```python
from build123d import *

# Parameters (mm, degrees)
ESQUISSE1_W                  = 90
ESQUISSE1_H                  = 25
BOSS_EXTRU_1_DEPTH           = 6
ESQUISSE2_W                  = 90
ESQUISSE2_H                  = 6
BOSS_EXTRU_2_DEPTH           = 40
ESQUISSE3_W                  = 40
ESQUISSE3_H                  = 6
BOSS_EXTRU_3_DEPTH           = 19
BOSS_EXTRU_4_DEPTH           = 6
ESQUISSE5_R                  = 2
ENL_V_MAT_EXTRU_1_DEPTH      = 157.783289926
ENL_V_MAT_EXTRU_2_DEPTH      = 160.25137362
ENL_V_MAT_EXTRU_2_DEPTH_BACK = 160.25137362
ESQUISSE6_R                  = 2
CHANFREIN1_SIZE              = 10
ESQUISSE7_R                  = 5
ENL_V_MAT_EXTRU_3_DEPTH      = 157.783289926
ESQUISSE8_R                  = 5
ENL_V_MAT_EXTRU_4_DEPTH      = 160.25137362
CHANFREIN3_SIZE              = 2.5
CONG_1_R                     = 10
CONG_2_R                     = 5


with BuildPart() as part:
    # Esquisse1 → Boss.-Extru.1 (new body)
    with BuildSketch(Plane.XY):
        with Locations((45, 12.5)):
            Rectangle(ESQUISSE1_W, ESQUISSE1_H)
    extrude(amount=BOSS_EXTRU_1_DEPTH)

    # Esquisse2 → Boss.-Extru.2 (add)
    with BuildSketch(Plane(origin=(90, 0, 0), x_dir=(0, 0, -1), z_dir=(1, 0, 0))):
        with Locations((-45, 3)):
            Rectangle(ESQUISSE2_W, ESQUISSE2_H)
    extrude(amount=BOSS_EXTRU_2_DEPTH)

    # Esquisse3 → Boss.-Extru.3 (add)
    with BuildSketch(Plane(origin=(0, 6, 0), x_dir=(1, 0, 0), z_dir=(0, 1, 0))):
        with Locations((110, -3)):
            Rectangle(ESQUISSE3_W, ESQUISSE3_H)
    extrude(amount=BOSS_EXTRU_3_DEPTH)

    # Esquisse4 → Boss.-Extru.4 (add)
    with BuildSketch(Plane.XZ):
        Polygon((0, 6), (90, 90), (90, 6), align=None)
    extrude(amount=-BOSS_EXTRU_4_DEPTH)

    # Esquisse5 → Enlèv. mat.-Extru.1 (cut, through all)
    with BuildSketch(Plane.XY.offset(6)):
        with Locations((45, 15.5)):
            Circle(ESQUISSE5_R)
        with Locations((15, 15.5)):
            Circle(ESQUISSE5_R)
        with Locations(Location((75, 15.5, 0), (0, 0, 180))):
            Circle(ESQUISSE5_R)
    extrude(amount=-ENL_V_MAT_EXTRU_1_DEPTH, mode=Mode.SUBTRACT)

    # Esquisse6 → Enlèv. mat.-Extru.2 (cut, two sides: drawn at the far end of the back side and taken through both)
    with BuildSketch(Plane(origin=(0, 6, 0), x_dir=(1, 0, 0), z_dir=(0, 1, 0)).offset(-ENL_V_MAT_EXTRU_2_DEPTH_BACK)):
        with Locations(Location((110, -48, 0), (0, 0, 270))):
            Circle(ESQUISSE6_R)
        with Locations(Location((110, -18, 0), (0, 0, 270))):
            Circle(ESQUISSE6_R)
        with Locations(Location((110, -78, 0), (0, 0, 90))):
            Circle(ESQUISSE6_R)
    extrude(amount=ENL_V_MAT_EXTRU_2_DEPTH + ENL_V_MAT_EXTRU_2_DEPTH_BACK, mode=Mode.SUBTRACT)

    # Chanfrein1
    # the kernel refuses this chamfer: 10 mm, written as the material it adds along each edge
    with BuildSketch(Plane(origin=(0, 6, 6), x_dir=(0, 0.9996219169112968, -0.027495876610586403), z_dir=(1, 0, 0))) as chanfrein1_piece_1_section:
        Polygon((CHANFREIN1_SIZE * 0.999621916911, CHANFREIN1_SIZE * 0.0274958766106), (-CHANFREIN1_SIZE * 0.0274958766106, CHANFREIN1_SIZE * 0.999621916911), (0, 0), align=None)
    chanfrein1_piece_1 = extrude(amount=130, mode=Mode.PRIVATE)
    chanfrein1_piece_1 = split(chanfrein1_piece_1, bisect_by=Plane(origin=(37.357692618, 9.297592043, 40.867179777), z_dir=(0.6823182503600111, 0, -0.7310552682428691)), keep=Keep.TOP, mode=Mode.PRIVATE)
    chanfrein1_piece_1 = chanfrein1_piece_1 - Plane(origin=(110, 9.297592043, 18), x_dir=(0, 0, 1), z_dir=(0, 1, 0)) * Cylinder(2, 300, mode=Mode.PRIVATE)
    chanfrein1_piece_1 = chanfrein1_piece_1 - Plane(origin=(15, 15.5, 9.259179561), x_dir=(1, 0, 0), z_dir=(0, 0, 1)) * Cylinder(2, 300, mode=Mode.PRIVATE)
    chanfrein1_piece_1 = chanfrein1_piece_1 - Plane(origin=(45, 15.5, 9.259179561), x_dir=(1, 0, 0), z_dir=(0, 0, 1)) * Cylinder(2, 300, mode=Mode.PRIVATE)
    chanfrein1_piece_1 = chanfrein1_piece_1 - Plane(origin=(75, 15.5, 9.259179561), x_dir=(-1, 0, 0), z_dir=(0, 0, 1)) * Cylinder(2, 300, mode=Mode.PRIVATE)
    add(chanfrein1_piece_1)

    # Esquisse7 → Enlèv. mat.-Extru.3 (cut, through all)
    with BuildSketch(Plane.XY.offset(6)):
        with Locations((45, 15.5)):
            Circle(ESQUISSE7_R)
        with Locations((15, 15.5)):
            Circle(ESQUISSE7_R)
        with Locations((75, 15.5)):
            Circle(ESQUISSE7_R)
    extrude(amount=ENL_V_MAT_EXTRU_3_DEPTH, mode=Mode.SUBTRACT)

    # Esquisse8 → Enlèv. mat.-Extru.4 (cut, through all)
    with BuildSketch(Plane(origin=(0, 6, 0), x_dir=(1, 0, 0), z_dir=(0, 1, 0))):
        with Locations((110, -18)):
            Circle(ESQUISSE8_R)
    extrude(amount=ENL_V_MAT_EXTRU_4_DEPTH, mode=Mode.SUBTRACT)

    # Chanfrein3
    chanfrein3_edges = [part.edges().sort_by_distance(p)[0] for p in [
        (43, 15.5, 6),
        (13, 15.5, 6),
        (77, 15.5, 6),
        (110, 6, 46),
        (110, 6, 16),
        (110, 6, 80),
    ]]
    chamfer(chanfrein3_edges, length=CHANFREIN3_SIZE)

    # Congé1
    cong_1_edges = [part.edges().sort_by_distance(p)[0] for p in [
        (90, 3, 90),
        (130, 3, 90),
    ]]
    fillet(cong_1_edges, radius=CONG_1_R)

    # Congé2
    cong_2_edges = [part.edges().sort_by_distance(p)[0] for p in [
        (130, 25, 3),
        (0, 25, 3),
        (0, 0, 3),
    ]]
    fillet(cong_2_edges, radius=CONG_2_R)


solid = part.part
```
CAD build for the part. Positions are in the model's coordinates, mm. A direction names the side the tool comes from. Round coordinates to 2 decimals unless told otherwise and drop trailing zeros. Write each loop counter-clockwise with the first axis right and the second up, starting at its lowest first coordinate (ties: lowest second). Pieces come first, ordered by that corner, then holes. Notation, with made-up numbers: M 6,89.25 L 37,89.25 A12 cw 37,109.25 Z; hole C 40,70 d3. An arc over 180 degrees is marked long. One line per question, with ' | ' between items.
1. Which spindle directions (+Z, -Z, +X, -X, +Y, -Y) get a long thin tool onto all of the face, cutting with end or side? Do faces 5 (the cylindrical face through (2, 1, 4)), 6 (the cylindrical face through (110, 7, 13)). Say none if no direction does.
Working result:
face 5: +Z, -Z, -X, -Y | face 6: +Z, +Y
2. Pin check, flat tips, straight feed: pin 1 Ø4.5 at (x, y) = (45, 15.5) entering from +Z; pin 2 Ø13 at (x, y) = (75, 15.5) entering from -Z; pin 3 Ø6.5 at (x, y) = (15, 15.5) entering from +Z; pin 4 Ø1 at (x, z) = (90.5, 62) entering from +Y. Stop position of each tip, or through.
Working result:
pin 1: z = 3.75 | pin 2: z = 0 | pin 3: z = 4.75 | pin 4: y = 6
3. Cut at B-B on z = 48. Write the cut outline in (x, y), and give its area (3 significant figures).
Working result:
outline: M 45,0 L 108,0 L 108,3.5 L 105.5,6 L 45,6 Z; M 112,0 L 130,0 L 130,6 L 114.5,6 L 112,3.5 Z | area: 480 mm2
4. Cut at A-A on x = 45. Write the cut outline in (y, z), and give its area (3 significant figures).
Working result:
outline: M 0,0 L 13.5,0 L 13.5,3.5 L 11,6 L 10.5,6 L 10.5,11.5 L 6,16 L 6,48 L 0,48 Z; M 17.5,0 L 25,0 L 25,6 L 20,6 L 17.5,3.5 Z | area: 407 mm2
5. Mould opens along Z. For faces 1 (the flat face through (64, 12, 0)), 2 (the conical face through (108.54, 3.66, 46.41)), 3 (the cylindrical face through (73.092, 14.899, 1.774)), 4 (the conical face through (46.96, 16.31, 3.62)) say: pulls with the +Z half, pulls with the -Z half, needs draft (parallel to the pull), parting line crosses it, or undercut.
Working result:
face 1: pulls with the -Z half | face 2: undercut | face 3: needs draft | face 4: pulls with the +Z half
6. Cut at C-C on x = 110. Write the cut outline in (y, z).
Working result:
outline: M 0,0 L 25,0 L 25,6 L 16,6 L 9,13 L 6,13 L 6,13.5 L 3.5,16 L 0,16 Z; M 0,20 L 3.5,20 L 6,22.5 L 6,43.5 L 3.5,46 L 0,46 Z; M 0,50 L 3.5,50 L 6,52.5 L 6,73.5 L 3.5,76 L 0,76 Z; M 0,80 L 3.5,80 L 6,82.5 L 6,90 L 0,90 Z
7. Cut at D-D on x = 65.5. Write the cut outline in (y, z), and give its area (3 significant figures).
Working result:
outline: M 0,0 L 25,0 L 25,6 L 16,6 L 6,16 L 6,67.13 L 0,67.13 Z | area: 567 mm2
8. Probe L1, parallel to X at y = 15.5, z = 0.7; L2, parallel to Z at x = 110, y = 1.4; L3, parallel to Y at x = 45, z = 2. List the from-to ranges inside material, lowest first. Write a range as from..to.
Working result:
L1: 0..13, 17..43, 47..73, 77..130 | L2: 0..16, 20..46, 50..76, 80..90 | L3: 0..13.5, 17.5..25
